For this review, take the finished solid that the model builds, in its own axes (mm). Give positions to 0.01 mm unless a question says otherwise; leave off trailing zeros.
```python
from build123d import *
from build123d import SkipClean  # not in build123d's __all__

# Parameters (mm, degrees)
F1_DEPTH = 20
F3_R     = 6.8
F3_R_2   = 6.5
F4_DEPTH = 20
F5_R     = 4.75
F6_DEPTH = 17


with BuildPart() as f1:
    # F0 (on Top) → F1 (new body)
    with BuildSketch(Plane.XY):
        with BuildLine():
            add(Edge.make_bspline(
                [(-34, 0), (-34.0019650757, 3.3683322836), (-8.8829017766, 21.2695751777), (13.7677686289, 10.092517361), (15, 0)],
                knots=[0, 0, 0, 0, 0.5, 1, 1, 1, 1], degree=3))
            Line((-34, 0), (-21.5, 0))
            ThreePointArc((-21.5, 0), (-15, 6.5), (-8.5, 0))
            Line((-8.5, 0), (-2.5, 0))
            ThreePointArc((-2.5, 0), (0, 2.5), (2.5, 0))
            Line((2.5, 0), (15, 0))
        make_face()
    extrude(amount=F1_DEPTH)

    # F2: F1 across plane


with BuildPart() as f1_1:
    add(f1.part, clean=False)
    with SkipClean():  # cleaning this boolean's faces spoils the solid; the shape is the same uncleaned
        add(f1.part.mirror(Plane.XZ), clean=False)

    # F3 (on Top) → F4 (join)
    with BuildSketch(Plane.XY):
        with Locations((-15, 0)):
            Circle(F3_R)
        with Locations((-15, 0)):
            Circle(F3_R_2, mode=Mode.SUBTRACT)
    with SkipClean():  # cleaning this boolean's faces spoils the solid; the shape is the same uncleaned
        extrude(amount=F4_DEPTH)


with BuildPart() as f6:
    # F5 (on Top) → F6 (new body)
    with BuildSketch(Plane.XY):
        Circle(F5_R)
    extrude(amount=F6_DEPTH)


with BuildPart() as f1_2:
    add(f1_1.part, clean=False)

    # F7: cut F6
    add(f6.part, mode=Mode.SUBTRACT)


solid = f1_2.part
```
Item 1: Take a section at A-A on y = -1.25. State how many separate pieces and enclosed holes the cut face has, and give its area (3 significant figures).
Answer:
separate pieces: 3
enclosed holes: 0
area: 544 mm2
Item 2: For L1, parallel to X at y = 0, z = 4.75; L2, parallel to X at y = -3, z = 15; L3, parallel to Y at x = 0, z = 9, list the stretches that pass through material, from the lowest coordinate up.
Answer:
L1: x = -34 to -21.5, -8.5 to -4.75, 4.75 to 15
L2: x = -32.22 to -20.77, -9.23 to -3.68, 3.68 to 14.3
L3: y = -13.8 to -4.75, 4.75 to 13.8
Item 3: Clearance check with flat-ended pins moving along their axes: pin 1 Ø5.5 at (x, y) = (0, 0) entering from +Z; pin 2 Ø5 at (y, z) = (-9.5, 14.5) entering from -X; pin 3 Ø5 at (y, z) = (6, 4) entering from +X; pin 4 Ø1.5 at (y, z) = (-11.5, 11) entering from +X. State where each tip first meets the part, or that it passes through.
Answer:
pin 1: stops at z = 20
pin 2: stops at x = -27.22
pin 3: stops at x = 14.11
pin 4: stops at x = 7.89
